```python
from build123d import *

# Parameters (mm, degrees)
SKETCH2_R                    = 150
BOSS_EXTRUDE1_DEPTH          = 75
CHAMFER1_SIZE                = 10
BOSS_EXTRUDE2_DEPTH          = 10
CHAMFER2_SIZE                = 7
BOSS_EXTRUDE3_DEPTH          = 9
BOSS_EXTRUDE4_DEPTH          = 3.5
CIRPATTERN1_COUNT            = 4
CIRPATTERN1_COPY_1_DEPTH     = 3.5
CIRPATTERN1_COPY_2_DEPTH     = 3.5
CIRPATTERN1_COPY_3_DEPTH     = 3.5
CIRPATTERN1_COPY_4_DEPTH     = 9
CIRPATTERN1_COPY_5_DEPTH     = 9
CIRPATTERN1_COPY_6_DEPTH     = 9
CHAMFER2_OF_CIRPATTERN1_SIZE = 7
CUT_EXTRUDE1_START           = -60
CUT_EXTRUDE1_DEPTH           = 60
SKETCH8_R                    = 110
BOSS_EXTRUDE5_DEPTH          = 9
BOSS_EXTRUDE5_TAPER          = 45
SKETCH9_R                    = 15
BOSS_EXTRUDE6_DEPTH          = 20


with BuildPart() as part:
    # Sketch2 → Boss-Extrude1 (new body)
    with BuildSketch(Plane(origin=(0, 0, 0), x_dir=(0, 0, -1), z_dir=(1, 0, 0))):
        Circle(SKETCH2_R)
    extrude(amount=BOSS_EXTRUDE1_DEPTH)

    # Chamfer1
    chamfer1_edges = [part.edges().sort_by_distance(p)[0] for p in [
        (75, 0, 150),
    ]]
    chamfer(chamfer1_edges, length=CHAMFER1_SIZE)

    # Sketch3 → Boss-Extrude2 (add)
    with BuildSketch(Plane.ZY):
        with BuildLine():
            Line((-37.5, 144.689485183), (-37.5, 194.689485183))
            Line((-37.5, 194.689485183), (37.5, 194.689485183))
            Line((37.5, 194.689485183), (37.5, 144.689485183))
            ThreePointArc((37.5, 144.689485183), (0, 149.470054267), (-37.5, 144.689485183))
        make_face()
    boss_extrude2 = extrude(amount=-BOSS_EXTRUDE2_DEPTH)

    # Chamfer2
    chamfer2_edges = [part.edges().sort_by_distance(p)[0] for p in [
        (5, 194.689485183, 37.5),
        (5, 194.689485183, -37.5),
    ]]
    chamfer(chamfer2_edges, length=CHAMFER2_SIZE)

    # Sketch4 → Boss-Extrude3 (add)
    with BuildSketch(Plane(origin=(0, 0, -37.5), x_dir=(-1, 0, 0), z_dir=(0, 0, -1))):
        Polygon((-10, 145.236875483), (-10, 187.689485183), (-65, 170.556875483), (-65, 145.236875483), align=None)
    boss_extrude3 = extrude(amount=-BOSS_EXTRUDE3_DEPTH)

    # Sketch5 → Boss-Extrude4 (add)
    with BuildSketch(Plane(origin=(10, 0, 0), x_dir=(0, 0, -1), z_dir=(1, 0, 0))):
        Polygon((21, 187.689485183), (18, 192.885637605), (12, 192.885637605), (9, 187.689485183), (12, 182.49333276), (18, 182.49333276), align=None)
    boss_extrude4 = extrude(amount=BOSS_EXTRUDE4_DEPTH)

    # Mirror1: Boss-Extrude4 across plane
    add(boss_extrude4.mirror(Plane.XY))

    # Mirror2: Boss-Extrude3 across plane
    add(boss_extrude3.mirror(Plane.XY))

    # CirPattern1: Boss-Extrude2, Boss-Extrude3, Boss-Extrude4 ×4 about axis
    cirpattern1_axis = Axis((0, 0, 0), (1, 0, 0))
    add([boss_extrude2.rotate(cirpattern1_axis, i * 360 / CIRPATTERN1_COUNT) for i in range(1, CIRPATTERN1_COUNT)])
    add([boss_extrude3.rotate(cirpattern1_axis, i * 360 / CIRPATTERN1_COUNT) for i in range(1, CIRPATTERN1_COUNT)])
    add([boss_extrude4.rotate(cirpattern1_axis, i * 360 / CIRPATTERN1_COUNT) for i in range(1, CIRPATTERN1_COUNT)])

    # CirPattern1 copy 1 sketch → CirPattern1 copy 1 (add)
    with BuildSketch(Plane(origin=(10, 0, 0), x_dir=(0, -1, 0), z_dir=(1, 0, 0))):
        Polygon((21, -187.689485183), (18, -192.885637605), (12, -192.885637605), (9, -187.689485183), (12, -182.49333276), (18, -182.49333276), align=None)
    extrude(amount=CIRPATTERN1_COPY_1_DEPTH)

    # CirPattern1 copy 2 sketch → CirPattern1 copy 2 (add)
    with BuildSketch(Plane(origin=(10, 0, 0), x_dir=(0, 0, -1), z_dir=(1, 0, 0))):
        Polygon((21, -187.689485183), (18, -192.885637605), (12, -192.885637605), (9, -187.689485183), (12, -182.49333276), (18, -182.49333276), align=None)
    extrude(amount=CIRPATTERN1_COPY_2_DEPTH)

    # CirPattern1 copy 3 sketch → CirPattern1 copy 3 (add)
    with BuildSketch(Plane.YZ.offset(10)):
        Polygon((21, -187.689485183), (18, -192.885637605), (12, -192.885637605), (9, -187.689485183), (12, -182.49333276), (18, -182.49333276), align=None)
    extrude(amount=CIRPATTERN1_COPY_3_DEPTH)

    # CirPattern1 copy 4 sketch → CirPattern1 copy 4 (add)
    with BuildSketch(Plane(origin=(0, -37.5, 0), x_dir=(-1, 0, 0), z_dir=(0, -1, 0))):
        Polygon((-10, -145.236875483), (-10, -187.689485183), (-65, -170.556875483), (-65, -145.236875483), align=None)
    extrude(amount=-CIRPATTERN1_COPY_4_DEPTH)

    # CirPattern1 copy 5 sketch → CirPattern1 copy 5 (add)
    with BuildSketch(Plane(origin=(0, 0, -37.5), x_dir=(-1, 0, 0), z_dir=(0, 0, -1))):
        Polygon((-10, -145.236875483), (-10, -187.689485183), (-65, -170.556875483), (-65, -145.236875483), align=None)
    extrude(amount=-CIRPATTERN1_COPY_5_DEPTH)

    # CirPattern1 copy 6 sketch → CirPattern1 copy 6 (add)
    with BuildSketch(Plane(origin=(0, 37.5, 0), x_dir=(-1, 0, 0), z_dir=(0, 1, 0))):
        Polygon((-10, -145.236875483), (-10, -187.689485183), (-65, -170.556875483), (-65, -145.236875483), align=None)
    extrude(amount=-CIRPATTERN1_COPY_6_DEPTH)

    # Chamfer2 of CirPattern1
    chamfer2_of_cirpattern1_edges = [part.edges().sort_by_distance(p)[0] for p in [
        (5, -37.5, 194.689485183),
        (5, 37.5, 194.689485183),
        (5, -194.689485183, -37.5),
        (5, -194.689485183, 37.5),
        (5, 37.5, -194.689485183),
        (5, -37.5, -194.689485183),
    ]]
    chamfer(chamfer2_of_cirpattern1_edges, length=CHAMFER2_OF_CIRPATTERN1_SIZE)

    # Sketch7 → Cut-Extrude1 (cut)
    with BuildSketch(Plane(origin=(75, 0, 0), x_dir=(0, 0, -1), z_dir=(1, 0, 0)).offset(CUT_EXTRUDE1_START)):
        with BuildLine():
            ThreePointArc((-70, -121.24355653), (-98.994949366, -98.994949366), (-121.24355653, -70))
            Line((-121.24355653, -70), (-129.903810568, -75))
            ThreePointArc((-129.903810568, -75), (-106.066017178, -106.066017178), (-75, -129.903810568))
            Line((-75, -129.903810568), (-70, -121.24355653))
        make_face()
        with BuildLine():
            ThreePointArc((-65, -112.583302492), (-91.923881554, -91.923881554), (-112.583302492, -65))
            Line((-112.583302492, -65), (-121.24355653, -70))
            ThreePointArc((-121.24355653, -70), (-98.994949366, -98.994949366), (-70, -121.24355653))
            Line((-70, -121.24355653), (-65, -112.583302492))
        make_face()
    extrude(amount=CUT_EXTRUDE1_DEPTH, mode=Mode.SUBTRACT)

    # Sketch8 → Boss-Extrude5 (add)
    with BuildSketch(Plane(origin=(75, 0, 0), x_dir=(0, 0, -1), z_dir=(1, 0, 0))):
        Circle(SKETCH8_R)
    extrude(amount=BOSS_EXTRUDE5_DEPTH, taper=BOSS_EXTRUDE5_TAPER)

    # Sketch9 → Boss-Extrude6 (add)
    with BuildSketch(Plane(origin=(84, 0, 0), x_dir=(0, 0, -1), z_dir=(1, 0, 0))):
        Circle(SKETCH9_R)
    extrude(amount=BOSS_EXTRUDE6_DEPTH)


solid = part.part
```
Could you check a few things on this model? Use its own coordinates, in mm. A direction names the side the tool comes from. Coordinates: 2 decimals unless noted, no trailing zeros. Write each loop counter-clockwise with the first axis right and the second up, starting at its lowest first coordinate (ties: lowest second). Pieces come first, ordered by that corner, then holes. Notation, with made-up numbers: (18.5, -12) -> (53.5, -12) arc R14 cw to (53.5, 13) -> close; hole circle Ø11 at (1, -17). An arc over 180 degrees is marked (long way). One line per question, with ' | ' between items. Start each with the question number.
1. For faces 4 (the face through (32, -37.5, 161)), 5 (the face through (38, -28.5, -163)), 6 (the face through (13.5, -188, -15)), 7 (the face through (75, 104, -41)), which set-ups out of +Z, -Z, +X, -X, +Y, -Y let a thin tool reach every point of the face, with its end or its side?
2. Will these pins go through, and if not, where does the flat tip stop? P1, Ø4, axis at x = 78, y = 13, coming from the +Z side; P2, Ø12, axis at x = 32.5, y = -159.5, coming from the -Z side; P3, Ø1, axis at x = 11, y = 15.5, coming from the +Z side.
3. If we section it at A-A (z = 0): Please give me the cut outline in (x, y).
4. Thinking about a two-plate mould opening in Y: for faces 1 (the face through (32.045, -106.854, -105.272)), 2 (the face through (38, 28.5, 163)), 3 (the face through (65, 33, 158)), which applies, pulls with the +Y half, pulls with the -Y half, needs draft (parallel to the pull), parting line crosses it, or undercut?
5. Please list where these lines run through material, in increasing order: line 1 along Y through (x, z) = (60, 167); line 2 along X through (y, z) = (90, -84); line 3 along Z through (x, y) = (40, 4).
Return value:
1) face 4: +Z, +X, -X, -Y | face 5: -Z, +X | face 6: +X, -Y | face 7: +X
2) P1: stops at z = 108.24 | P2: stops at z = -37.5 | P3: stops at z = 192.89
3) outline: (0, -194.69) -> (10, -194.69) -> (10, -150) -> (65, -150) -> (75, -140) -> (75, -110) -> (84, -101) -> (84, -15) -> (104, -15) -> (104, 15) -> (84, 15) -> (84, 101) -> (75, 110) -> (75, 140) -> (65, 150) -> (10, 150) -> (10, 194.69) -> (0, 194.69) -> close
4) face 1: pulls with the -Y half | face 2: undercut | face 3: needs draft
5) line 1: y = -37.5 to -28.5, 28.5 to 37.5 | line 2: x = 0 to 75 | line 3: z = -149.95 to 149.95
